Input: part model. Units: mm. Frame: model coordinates. Face numbers are marked on the shaded views. Give positions to 0.01 mm unless a question says otherwise; leave off trailing zeros. Order: outer loops, then holes, each group sorted by start corner. A loop starts at its lowest first (then second) coordinate and runs counter-clockwise, first axis right, second up. Notation, with made-up numbers: (-18, 73) -> (11, 73) arc R26 ccw to (11, 99) -> close; hole circle Ø8 at (66.25, 46.5). An arc over 180 degrees is marked (long way). Use a Markdown table: item, result. Add a question column.
from build123d import *

# Parameters (mm, degrees)
F0_W          = 110
F0_H          = 90
F1_DEPTH      = 75
F2_T          = 3
F4_DEPTH      = 25.4
F5_W          = 3
F5_H          = 60
F6_DEPTH      = 110
F8_DEPTH      = 76
F8_DEPTH_BACK = 88
F9_R          = 5


with BuildPart() as f1:
    # F0 (on Top) → F1 (new body, symmetric)
    with BuildSketch(Plane.XY):
        Rectangle(F0_W, F0_H)
    extrude(amount=F1_DEPTH, both=True)

    # F2
    f2_openings = [f1.faces().sort_by_distance(p)[0] for p in [
        (0, 0, -75),
    ]]
    offset(amount=F2_T, openings=f2_openings, kind=Kind.INTERSECTION)

    # F3 (on face) → F4 (cut)
    with BuildSketch(Plane.YZ.offset(58)):
        with BuildLine():
            Line((0, 55), (0, 75))
            ThreePointArc((0, 75), (-7.0710678119, 72.0710678119), (-10, 65))
            ThreePointArc((-10, 65), (-7.0710678119, 57.9289321881), (0, 55))
        make_face()
        with BuildLine():
            ThreePointArc((10, 65), (7.0710678119, 72.0710678119), (0, 75))
            Line((0, 75), (0, 55))
            ThreePointArc((0, 55), (7.0710678119, 57.9289321881), (10, 65))
        make_face()
    extrude(amount=-F4_DEPTH, mode=Mode.SUBTRACT)

    # F5 (on face) → F6 (join)
    with BuildSketch(Plane(origin=(55, 0, 0), x_dir=(0, -1, 0), z_dir=(-1, 0, 0))):
        with Locations((-23.5, 48)):
            Rectangle(F5_W, F5_H)
    extrude(amount=F6_DEPTH)

    # F7 (on face) → F8 (cut, two sides)
    with BuildSketch(Plane(origin=(0, -45, 0), x_dir=(-1, 0, 0), z_dir=(0, 1, 0))) as f8_sk:
        with BuildLine():
            ThreePointArc((3, 30), (-2.1213203436, 32.1213203436), (0, 27))
            ThreePointArc((0, 27), (2.1213203436, 27.8786796564), (3, 30))
        make_face()
    extrude(amount=-F8_DEPTH, mode=Mode.SUBTRACT)
    extrude(f8_sk.sketch, amount=F8_DEPTH_BACK, mode=Mode.SUBTRACT)

    # F9
    f9_edges = [f1.edges().sort_by_distance(p)[0] for p in [
        (-58, 48, 1.5),
        (-58, -48, 1.5),
    ]]
    fillet(f9_edges, radius=F9_R)


solid = f1.part
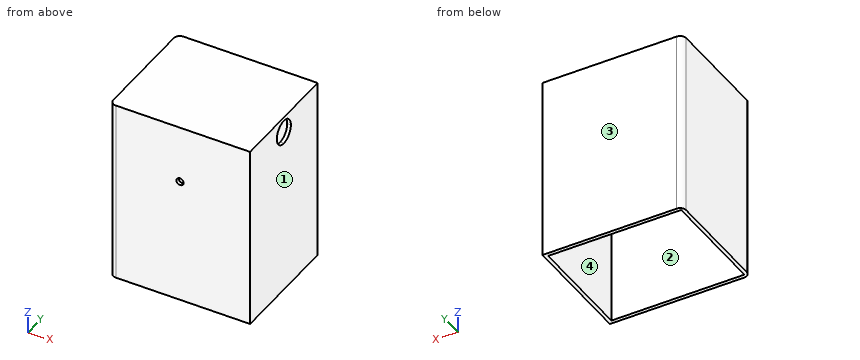
Q1. Section query C-C (x = -35). Return loops of the section in (y, z), plus the area to 3 significant figures.
Q2. Section query D-D (y = -39.5). Return loops of the section in (x, z).
Q3. First-contact query: pin 1 (16 mm diameter, centred on x = -8, y = 35.5, fed in from -Z); pin 2 (5.5 mm diameter, centred on x = 0, z = 30, fed in from -Y); pin 3 (2.5 mm diameter, centred on x = 10, y = 23, fed in from -Z); pin 4 (8 mm diameter, centred on x = 0, z = 30, fed in from -Y). Flat tips, straight axial feed; report the tip coordinate or a pass-through.
Q4. Section query B-B (y = 4). Return loops of the section in (x, z), plus the area to 3 significant figures.
Q5. Ray query, line 1 (Y direction, x = -45, z = 21); line 2 (Y direction, x = -16, z = -41.5); line 3 (X direction, y = -25, z = -17.5). Return the intervals inside material, ascending.
Q6. Section query A-A (z = 9.5). Return loops of the section in (x, y), plus the area to 3 significant figures.
Q7. Draft query along X for the marked faces 1, 2, 3 and 4. Return one class per face: +X half, -X half, draft (parallel to the pull), parting line (faces both ways), or undercut.
Solution:
| question | item | result |
|---|---|---|
| 1 | outline | (-48, -75) -> (-45, -75) -> (-45, 75) -> (22, 75) -> (22, 18) -> (25, 18) -> (25, 75) -> (45, 75) -> (45, -75) -> (48, -75) -> (48, 78) -> (-48, 78) -> close |
| 1 | area | 1,360 mm² |
| 2 | outline | (-58, -75) -> (-55, -75) -> (-55, 75) -> (55, 75) -> (55, -75) -> (58, -75) -> (58, 78) -> (-58, 78) -> close |
| 3 | pin 1 | stops at z = 75 |
| 3 | pin 2 | stops at y = 45 |
| 3 | pin 3 | stops at z = 18 |
| 3 | pin 4 | stops at y = -48 |
| 4 | outline | (-58, -75) -> (-55, -75) -> (-55, 75) -> (55, 75) -> (55, 74.17) -> (58, 74.17) -> (58, 78) -> (-58, 78) -> close; (55, -75) -> (58, -75) -> (58, 55.83) -> (55, 55.83) -> close |
| 4 | area | 1,190 mm² |
| 5 | line 1 | y = -48 to -45, 22 to 25, 45 to 48 |
| 5 | line 2 | y = -48 to -45, 45 to 48 |
| 5 | line 3 | x = -58 to -55, 55 to 58 |
| 6 | outline | (-58, -43) arc R5 ccw to (-53, -48) -> (58, -48) -> (58, 48) -> (-53, 48) arc R5 ccw to (-58, 43) -> close; hole (-55, -45) -> (55, -45) -> (55, 45) -> (-55, 45) -> close |
| 6 | area | 1,230 mm² |
| 7 | face 1 | +X half |
| 7 | face 2 | undercut |
| 7 | face 3 | draft |
| 7 | face 4 | undercut |
